Here's the drawing with two shaded views (mm, measured from the low corner). I have some questions. A direction names the side the tool comes from. Coordinates: 2 decimals unless noted, no trailing zeros. Loops run counter-clockwise (first coordinate to the right, second up) from the corner with the lowest first, then second, coordinate; pieces in that order, holes last. Notation, with made-up numbers: (1.25, 84.25) - (37.25, 84.25) arc R23 cw to (37.25, 102.25) - close; hole circle Ø5 at (14, 9). An arc over 180 degrees is marked (long way). Use a Markdown table: item, result.
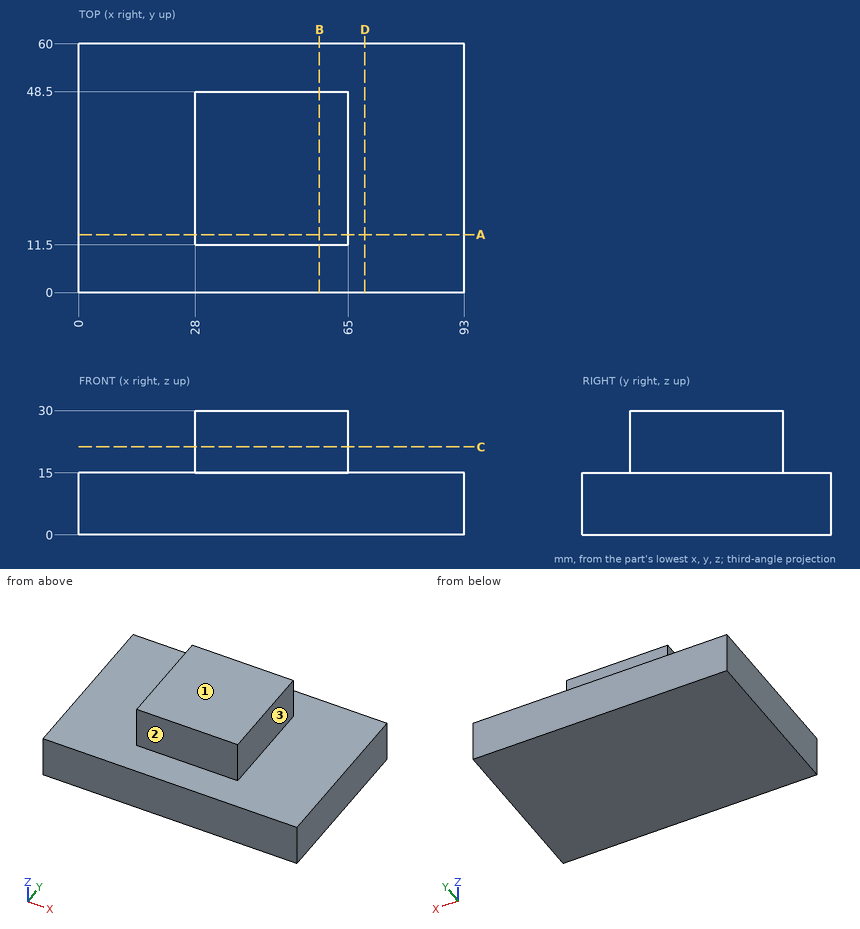
Q1. I want a section at A-A, the plane y = 14. Write out the boundary of the cut face in (x, z), then the cut area to 3 significant figures.
Check values:
| item | result |
|---|---|
| outline | (0, 0) - (93, 0) - (93, 15) - (65, 15) - (65, 30) - (28, 30) - (28, 15) - (0, 15) - close |
| area | 1,950 mm^2 |
Q2. Which directions (+Z, -Z, +X, -X, +Y, -Y) give clear straight access to the entire face, cutting with the end or side of a thin tool? Please do the marked faces 1, 2 and 3.
Check values:
| item | result |
|---|---|
| face 1 | +Z, +X, -X, +Y, -Y |
| face 2 | +Z, +X, -X, -Y |
| face 3 | +Z, +X, +Y, -Y |
Q3. I want a section at C-C, the plane z = 21.25. Write out the boundary of the cut face in (x, y), then the cut area to 3 significant figures.
Check values:
| item | result |
|---|---|
| outline | (28, 11.5) - (65, 11.5) - (65, 48.5) - (28, 48.5) - close |
| area | 1,370 mm^2 |
Q4. Will these pins go through, and if not, where does the flat tip stop? P1, Ø12, axis at x = 32, z = 25.5, coming from the +Y side; P2, Ø7.5, axis at y = 21.5, z = 26, coming from the +X side; P3, Ø4, axis at x = 79, y = 34, coming from the -Z side; P4, Ø16.5, axis at x = 43, z = 24, coming from the -Y side.
Check values:
| item | result |
|---|---|
| P1 | y = 48.5 |
| P2 | x = 65 |
| P3 | z = 0 |
| P4 | y = 11.5 |
Q5. Please list where these lines run through material, in increasing order: L1, parallel to Y at x = 35, z = 29; L2, parallel to X at y = 40, z = 26.75; L3, parallel to Z at x = 17.5, y = 14.5. Write a range as from..to.
Check values:
| item | result |
|---|---|
| L1 | 11.5..48.5 |
| L2 | 28..65 |
| L3 | 0..15 |
Q6. I want a section at B-B, the plane x = 58. Write out the boundary of the cut face in (y, z), then the cut area to 4 significant figures.
Check values:
| item | result |
|---|---|
| outline | (0, 0) - (60, 0) - (60, 15) - (48.5, 15) - (48.5, 30) - (11.5, 30) - (11.5, 15) - (0, 15) - close |
| area | 1,455 mm^2 |
Q7. I want a section at D-D, the plane x = 69. Write out the boundary of the cut face in (y, z), then the cut area to 3 significant figures.
Check values:
| item | result |
|---|---|
| outline | (0, 0) - (60, 0) - (60, 15) - (0, 15) - close |
| area | 900 mm^2 |
